```python
from build123d import *

# Parameters (mm, degrees)
SKETCH1_W           = 20
SKETCH1_H           = 8
SKETCH1_R           = 2.2
SKETCH1_R_2         = 2.25
SKETCH1_R_3         = 2.3
BOSS_EXTRUDE1_DEPTH = 5
FILLET1_R           = 2


with BuildPart() as part:
    # Sketch1 → Boss-Extrude1 (new body)
    with BuildSketch(Plane(origin=(0, 0, 0), x_dir=(1, 0, 0), z_dir=(0, 1, 0))):
        Rectangle(SKETCH1_W, SKETCH1_H)
        with Locations((-6, 0)):
            Circle(SKETCH1_R, mode=Mode.SUBTRACT)
        Circle(SKETCH1_R_2, mode=Mode.SUBTRACT)
        with Locations((6, 0)):
            Circle(SKETCH1_R_3, mode=Mode.SUBTRACT)
    extrude(amount=BOSS_EXTRUDE1_DEPTH)

    # Fillet1
    fillet1_edges = [part.edges().sort_by_distance(p)[0] for p in [
        (10, 2.5, 4),
        (-10, 2.5, 4),
        (-10, 2.5, -4),
        (10, 2.5, -4),
    ]]
    fillet(fillet1_edges, radius=FILLET1_R)


solid = part.part
```
Geometry: final body of the model. Coordinates: model frame, mm. Give positions to 0.01 mm unless a question says otherwise; leave off trailing zeros. Loops run counter-clockwise (first coordinate to the right, second up) from the corner with the lowest first, then second, coordinate; pieces in that order, holes last. Notation, with made-up numbers: (61.5, 88.25) - (113.5, 88.25) arc R17 ccw to (113.5, 110.25) - close; hole circle Ø2 at (59.25, -5). An arc over 180 degrees is marked (long way). Answer as CSV lines item,"result". Start each with the question number.
(1) Section query A-A (x = 0). Output: boundary loops of the cut face in (y, z), and give its area (3 significant figures).
(2) Ray query, line 1 along X through (y, z) = (3.05, 0); line 2 along Z through (x, y) = (-6, 3.2); line 3 along X through (y, z) = (3.5, 1.5). Return the intervals inside material, ascending. Write a range as [from, to].
(3) Section query B-B (z = 0). Output: boundary loops of the cut face in (x, y).
(4) Mould query, pull axis Z, two halves, no side actions, for faces 1 (the face through (-9.43, 2.54, 3.4)), 2 (the face through (-9.43, 2.54, -3.4)), 3 (the face through (-0.29, 2.46, -2.23)). Classes: +Z half, -Z half, draft (parallel to the pull), parting line (faces both ways), or undercut.
(5) Section query D-D (x = 6). Output: boundary loops of the cut face in (y, z), and give its area (3 significant figures).
(6) Section query C-C (y = 4.6). Output: boundary loops of the cut face in (x, z).
Worked answers:
1,outline,"(0, -4) - (5, -4) - (5, -2.25) - (0, -2.25) - close; (0, 2.25) - (5, 2.25) - (5, 4) - (0, 4) - close"
1,area,"17.5 mm^2"
2,line 1,"x = [-10, -8.2], [-3.8, -2.25], [2.25, 3.7], [8.3, 10]"
2,line 2,"z = [-4, -2.2], [2.2, 4]"
2,line 3,"x = [-10, -7.61], [-4.39, -1.68], [1.68, 4.26], [7.74, 10]"
3,outline,"(-10, 0) - (-8.2, 0) - (-8.2, 5) - (-10, 5) - close; (-3.8, 0) - (-2.25, 0) - (-2.25, 5) - (-3.8, 5) - close; (2.25, 0) - (3.7, 0) - (3.7, 5) - (2.25, 5) - close; (8.3, 0) - (10, 0) - (10, 5) - (8.3, 5) - close"
4,face 1,"+Z half"
4,face 2,"-Z half"
4,face 3,"undercut"
5,outline,"(0, -4) - (5, -4) - (5, -2.3) - (0, -2.3) - close; (0, 2.3) - (5, 2.3) - (5, 4) - (0, 4) - close"
5,area,"17.0 mm^2"
6,outline,"(-10, -2) arc R2 ccw to (-8, -4) - (8, -4) arc R2 ccw to (10, -2) - (10, 2) arc R2 ccw to (8, 4) - (-8, 4) arc R2 ccw to (-10, 2) - close; hole circle Ø4.4 at (-6, 0); hole circle Ø4.5 at (0, 0); hole circle Ø4.6 at (6, 0)"
